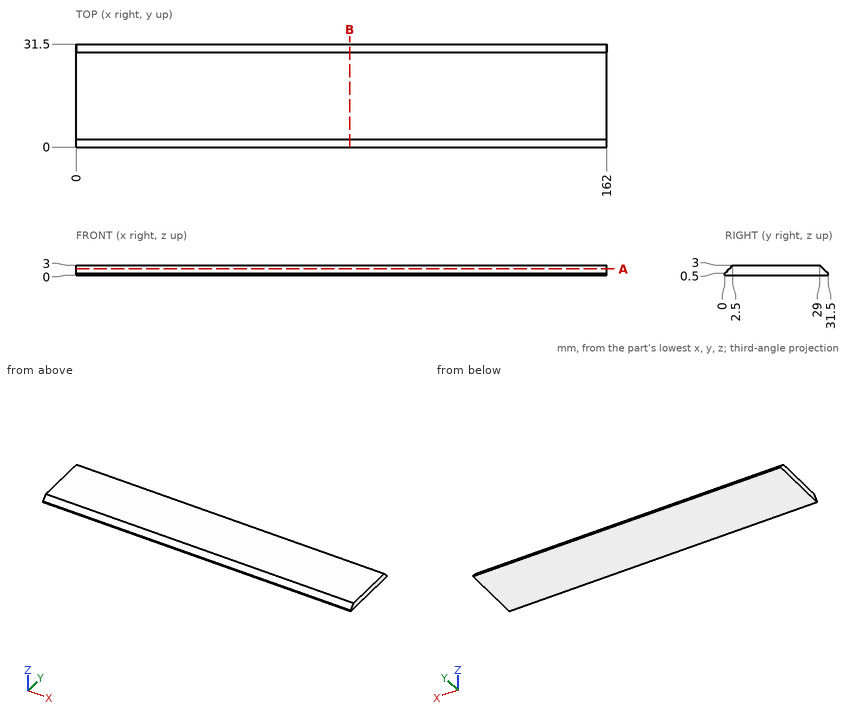
Could you check a few things on this drawing? It's one solid part, dimensions in mm from its lowest x, y, z. Give positions to 0.01 mm unless a question says otherwise; leave off trailing zeros. Order: outer loops, then holes, each group sorted by start corner. A loop starts at its lowest first (then second) coordinate and runs counter-clockwise, first axis right, second up.
1. Suppose I cut it at B-B (x = 83.5). Write out the boundary of the cut face in (y, z).
Answers below:
outline: (0, 0) - (31.5, 0) - (31.5, 0.5) - (29, 3) - (2.5, 3) - (0, 0.5) - close
2. Suppose I cut it at A-A (z = 1.9). Write out the boundary of the cut face in (x, y).
Answers below:
outline: (0, 1.4) - (162, 1.4) - (162, 30.1) - (0, 30.1) - close
3. I need wall thicknesses on L1, parallel to Z at x = 86, y = 29.5; L2, parallel to Y at x = 53, z = 2.55; L3, parallel to Y at x = 42.5, z = 2.75. Which ranges of each line are inside material? Lowest first, please.
Answers below:
L1: z = 0 to 2.5
L2: y = 2.05 to 29.45
L3: y = 2.25 to 29.25
